```python
from build123d import *

# Parameters (mm, degrees)
SKETCH1_W                = 127
SKETCH1_H                = 76.2
BOSS_EXTRUDE1_DEPTH      = 3.175
BOSS_EXTRUDE2_DEPTH      = 12.7
BOSS_EXTRUDE2_DEPTH_BACK = 25.4
SKETCH2_R                = 9.525
F_1_2_13_TAPPED_HOLE3_D  = 11.684
THREAD2_PITCH            = 1.953846154
THREAD2_HEIGHT           = 30.32
THREAD2_RADIUS           = 5.842
SKETCH12_R               = 1.905
CUT_EXTRUDE1_DEPTH       = 79.28805787
SKETCH13_R               = 9.525
CUT_EXTRUDE2_DEPTH       = 6.35
SKETCH15_R               = 9.525
CUT_EXTRUDE4_DEPTH       = 81.572467421


with BuildPart() as part:
    # Sketch1 → Boss-Extrude1 (new body)
    with BuildSketch(Plane.XY):
        Rectangle(SKETCH1_W, SKETCH1_H)
    extrude(amount=BOSS_EXTRUDE1_DEPTH)

    # Sketch2 → Boss-Extrude2 (add, two sides: drawn at the far end of the back side and taken through both)
    with BuildSketch(Plane.XY.offset(3.175).offset(-BOSS_EXTRUDE2_DEPTH_BACK)):
        Circle(SKETCH2_R)
    extrude(amount=BOSS_EXTRUDE2_DEPTH + BOSS_EXTRUDE2_DEPTH_BACK)

    # 1/2-13 Tapped Hole3 (through all)
    with Locations(Plane.XY.offset(15.875)):
        with Locations((0, 0)):
            Hole(F_1_2_13_TAPPED_HOLE3_D / 2)

    # Thread2: sweep along a helix
    with BuildLine() as thread2_path:
        Helix(THREAD2_PITCH, THREAD2_HEIGHT, THREAD2_RADIUS, center=(0, 0, 15.875), direction=(0, 0, -1))
    # Thread Profile2 → Thread2 (sweep)
    with BuildSketch(Plane(origin=(-5.842, 0, 15.875), x_dir=(-1, 0, 0), z_dir=(0, -1, 0))):
        Polygon((0, 0), (1.057550248, 0.61057692), (1.057550248, 0.85480769), (0, 1.46538461), align=None)
    sweep(path=thread2_path.line, is_frenet=True)

    # Sketch12 → Cut-Extrude1 (cut, through all)
    with BuildSketch(Plane.XY.offset(3.175)):
        with Locations((-38.1, 25.4)):
            Circle(SKETCH12_R)
        with Locations((-38.1, -25.4)):
            Circle(SKETCH12_R)
        with Locations((38.1, -25.4)):
            Circle(SKETCH12_R)
        with Locations((38.1, 25.4)):
            Circle(SKETCH12_R)
    extrude(amount=-CUT_EXTRUDE1_DEPTH, mode=Mode.SUBTRACT)

    # Sketch13 → Cut-Extrude2 (cut)
    with BuildSketch(Plane.XY.offset(15.875)):
        Circle(SKETCH13_R)
    extrude(amount=-CUT_EXTRUDE2_DEPTH, mode=Mode.SUBTRACT)

    # Sketch15 → Cut-Extrude4 (cut, through all)
    with BuildSketch(Plane.XY.offset(9.525)):
        Circle(SKETCH15_R)
    extrude(amount=-CUT_EXTRUDE4_DEPTH, mode=Mode.SUBTRACT)


solid = part.part
```
Design review of the part built by this model. Coordinates are the model's own, in mm. Give positions to 0.01 mm unless a question says otherwise; leave off trailing zeros. Loops run counter-clockwise (first coordinate to the right, second up) from the corner with the lowest first, then second, coordinate; pieces in that order, holes last. Notation, with made-up numbers: (-2, -24) -> (4, -24) arc R9 ccw to (4, -17) -> close; hole circle Ø7 at (53.25, 73). An arc over 180 degrees is marked (long way). Write each question's results on one line, items separated by ' | '.
Q1. The part is to be moulded in two halves that separate along X. For faces 1 (the face through (13, 1, 3.175)), 2 (the face through (39.917, 25.972, 1.61)), 3 (the face through (63.5, -1, 2)), say which applies: +X half, -X half, draft (parallel to the pull), parting line (faces both ways), or undercut.
Reply:
face 1: draft | face 2: undercut | face 3: +X half
Q2. Take a section at D-D, the plane x = 0. Write out the cut boundary in (y, z) (3 decimals), plus the area to 3 significant figures.
Reply:
outline: (-38.1, 0) -> (-9.525, 0) -> (-9.525, 3.175) -> (-38.1, 3.175) -> close; (9.525, 0) -> (38.1, 0) -> (38.1, 3.175) -> (9.525, 3.175) -> close | area: 181 mm²
Q3. Wall thickness on L1, parallel to Y at x = -38.1, z = 1.6 (3 decimals); L2, parallel to X at y = 0, z = 1.3 (3 decimals); L3, parallel to X at y = -2, z = 1.85: over which ranges is each line inside the solid? List them lowest first.
Reply:
L1: y = -38.1 to -27.305, -23.495 to 23.495, 27.305 to 38.1 | L2: x = -63.5 to -9.525, 9.525 to 63.5 | L3: x = -63.5 to -9.31, 9.31 to 63.5
Q4. Take a section at A-A, the plane x = -38.1. Write out the cut boundary in (y, z) (3 decimals), plus the area to 3 significant figures.
Reply:
outline: (-38.1, 0) -> (-27.305, 0) -> (-27.305, 3.175) -> (-38.1, 3.175) -> close; (-23.495, 0) -> (23.495, 0) -> (23.495, 3.175) -> (-23.495, 3.175) -> close; (27.305, 0) -> (38.1, 0) -> (38.1, 3.175) -> (27.305, 3.175) -> close | area: 218 mm²
Q5. Take a section at B-B, the plane z = 1. Write out the cut boundary in (x, y) (3 decimals).
Reply:
outline: (-63.5, -38.1) -> (63.5, -38.1) -> (63.5, 38.1) -> (-63.5, 38.1) -> close; hole circle Ø3.81 at (-38.1, -25.4); hole circle Ø3.81 at (-38.1, 25.4); hole circle Ø19.05 at (0, 0); hole circle Ø3.81 at (38.1, -25.4); hole circle Ø3.81 at (38.1, 25.4)
Q6. Take a section at C-C, the plane y = 0. Write out the cut boundary in (x, z) (3 decimals), plus the area to 3 significant figures.
Reply:
outline: (-63.5, 0) -> (-9.525, 0) -> (-9.525, 3.175) -> (-63.5, 3.175) -> close; (9.525, 0) -> (63.5, 0) -> (63.5, 3.175) -> (9.525, 3.175) -> close | area: 343 mm²
